from build123d import *

# Parameters (mm, degrees)
CROQUIS1_R              = 10
SALIENTE_EXTRUIR1_DEPTH = 25
CROQUIS2_R              = 20
SALIENTE_EXTRUIR2_DEPTH = 2
SALIENTE_EXTRUIR3_START = -25
CROQUIS2_2_R            = 20
SALIENTE_EXTRUIR3_DEPTH = 2
CROQUIS3_R              = 2.5
CORTAR_EXTRUIR1_DEPTH   = 26
CROQUIS4_R              = 0.5
CORTAR_EXTRUIR2_DEPTH   = 0.5
CORTAR_EXTRUIR3_START   = -25
CROQUIS4_2_R            = 0.5
CORTAR_EXTRUIR3_DEPTH   = 0.5


with BuildPart() as part:
    # Croquis1 → Saliente-Extruir1 (new body)
    with BuildSketch(Plane(origin=(0, 0, 0), x_dir=(1, 0, 0), z_dir=(0, 1, 0))):
        Circle(CROQUIS1_R)
    extrude(amount=SALIENTE_EXTRUIR1_DEPTH)

    # Croquis2 → Saliente-Extruir2 (add)
    with BuildSketch(Plane(origin=(0, 25, 0), x_dir=(1, 0, 0), z_dir=(0, 1, 0))):
        Circle(CROQUIS2_R)
    extrude(amount=-SALIENTE_EXTRUIR2_DEPTH)

    # Croquis2_2 → Saliente-Extruir3 (add)
    with BuildSketch(Plane(origin=(0, 25, 0), x_dir=(1, 0, 0), z_dir=(0, 1, 0)).offset(SALIENTE_EXTRUIR3_START)):
        Circle(CROQUIS2_2_R)
    extrude(amount=SALIENTE_EXTRUIR3_DEPTH)

    # Croquis3 → Cortar-Extruir1 (cut, through all)
    with BuildSketch(Plane(origin=(0, 25, 0), x_dir=(1, 0, 0), z_dir=(0, 1, 0))):
        Circle(CROQUIS3_R)
    extrude(amount=-CORTAR_EXTRUIR1_DEPTH, mode=Mode.SUBTRACT)

    # Croquis4 → Cortar-Extruir2 (cut)
    with BuildSketch(Plane(origin=(0, 25, 0), x_dir=(1, 0, 0), z_dir=(0, 1, 0))):
        with Locations((0, 5)):
            Circle(CROQUIS4_R)
        with Locations((5, 0)):
            Circle(CROQUIS4_R)
        with Locations((0, -5)):
            Circle(CROQUIS4_R)
        with Locations((-5, 0)):
            Circle(CROQUIS4_R)
    extrude(amount=-CORTAR_EXTRUIR2_DEPTH, mode=Mode.SUBTRACT)

    # Croquis4_2 → Cortar-Extruir3 (cut)
    with BuildSketch(Plane(origin=(0, 25, 0), x_dir=(1, 0, 0), z_dir=(0, 1, 0)).offset(CORTAR_EXTRUIR3_START)):
        with Locations((0, 5)):
            Circle(CROQUIS4_2_R)
        with Locations((5, 0)):
            Circle(CROQUIS4_2_R)
        with Locations((0, -5)):
            Circle(CROQUIS4_2_R)
        with Locations((-5, 0)):
            Circle(CROQUIS4_2_R)
    extrude(amount=CORTAR_EXTRUIR3_DEPTH, mode=Mode.SUBTRACT)


solid = part.part
Model file for the job. Use its own axes, mm. A direction names the side the tool comes from. Give positions to 0.01 mm unless a question says otherwise; leave off trailing zeros. Order: outer loops, then holes, each group sorted by start corner. A loop starts at its lowest first (then second) coordinate and runs counter-clockwise, first axis right, second up. Notation, with made-up numbers: (20, -38) -> (62, -38) arc R16 ccw to (62, -26) -> close; hole circle Ø11 at (13.25, 75). An arc over 180 degrees is marked (long way). Use CSV: the item, a comma, the result in double quotes.
1. Drill centre lines: line 1 along X through (y, z) = (24.6, 0); line 2 along Y through (x, z) = (-11, -14); line 3 along X through (y, z) = (24.8, 5). Where is each one in solid material? Low to high. Write a range as from..to.
Outcome:
line 1,"-20..-5.5, -4.5..-2.5, 2.5..4.5, 5.5..20"
line 2,"0..2, 23..25"
line 3,"-19.36..-0.5, 0.5..19.36"
2. Band-saw the part on C-C, the plane y = 23.75. Give the cut face in (x, z), then the cut area to 3 significant figures.
Outcome:
outline,"circle Ø40 at (0, 0); hole circle Ø5 at (0, 0)"
area,"1,240 mm²"
3. Drop flat-ended pins along their axis: pin 1 (1.5 mm diameter, centred on y = 5, z = -8, fed in from -X); pin 2 (0.8 mm diameter, centred on x = 0, z = -5, fed in from +Y); pin 3 (0.8 mm diameter, centred on x = -5, z = 0, fed in from -Y); pin 4 (6 mm diameter, centred on x = 13.5, y = 7.5, fed in from +Z). Give the stop position or say it passes through.
Outcome:
pin 1,"x = -6.89"
pin 2,"y = 24.5"
pin 3,"y = 0.5"
pin 4,"through"
4. Mould opens along Y. For faces 1 (the flat face through (-5, 23, -9)), 2 (the cylindrical face through (-0.065, 24.754, -5.496)), 3 (the flat face through (5, 0.5, 0)) say: +Y half, -Y half, draft (parallel to the pull), parting line (faces both ways), or undercut.
Outcome:
face 1,"undercut"
face 2,"draft"
face 3,"-Y half"
5. 3-axis set-ups, long thin cutter, end or side, ignore diameter. For faces 4 (the flat face through (4, 25, 0)), 5 (the cylindrical face through (-0.065, 0.246, -5.496)), 6 (the cylindrical face through (4.6, 24.8, 0.3)), 7 (the flat face through (-5, 2, -9)): which of +Z, -Z, +X, -X, +Y, -Y reach the whole face in a straight line?
Outcome:
face 4,"+Z, -Z, +X, -X, +Y"
face 5,"-Y"
face 6,"+Y"
face 7,"none"
6. Band-saw the part on A-A, the plane z = 16. Give the cut face in (x, y).
Outcome:
outline,"(-12, 0) -> (12, 0) -> (12, 2) -> (-12, 2) -> close; (-12, 23) -> (12, 23) -> (12, 25) -> (-12, 25) -> close"
